Input: part model. Units: mm. Frame: model coordinates. A direction names the side the tool comes from. Round coordinates to 2 decimals unless told otherwise and drop trailing zeros. Order: outer loops, then holes, each group sorted by start corner. A loop starts at its lowest first (then second) coordinate and runs counter-clockwise, first axis right, second up. Notation, with made-up numbers: (53, -3) - (58, -3) arc R23 ccw to (58, 30) - close; hole circle Ø9 at (63.25, -9). An arc over 180 degrees is marked (long way). One line per item, written item: value. Start each with the question number.
from build123d import *

# Parameters (mm, degrees)
SKIZZE1_R                       = 30
AUFSATZ_LINEAR_AUSTRAGEN1_DEPTH = 30
SKIZZE2_R                       = 7.5
AUFSATZ_LINEAR_AUSTRAGEN2_DEPTH = 40
KREISMUSTER1_COUNT              = 8


with BuildPart() as part:
    # Skizze1 → Aufsatz-Linear austragen1 (new body)
    with BuildSketch(Plane.XY):
        Circle(SKIZZE1_R)
    extrude(amount=AUFSATZ_LINEAR_AUSTRAGEN1_DEPTH)

    # Skizze2 → Aufsatz-Linear austragen2 (add)
    with BuildSketch(Plane(origin=(0, 0, 0), x_dir=(1, 0, 0), z_dir=(0, 1, 0))):
        with Locations(Location((0, -15, 0), (0, 0, 90))):
            Circle(SKIZZE2_R)
    aufsatz_linear_austragen2 = extrude(amount=AUFSATZ_LINEAR_AUSTRAGEN2_DEPTH)

    # Kreismuster1: Aufsatz-Linear austragen2 ×8 about axis
    kreismuster1_axis = Axis((0, 0, 0), (0, 0, 1))
    for i in range(1, KREISMUSTER1_COUNT):
        add(aufsatz_linear_austragen2.rotate(kreismuster1_axis, i * 360 / KREISMUSTER1_COUNT))


solid = part.part
Item 1: Pull-direction query (Y, two-part tool) for faces 1 (the face through (0, 40, 15)), 2 (the face through (0, -40, 15)), 3 (the face through (19.099, 29.616, 15.976)); classes: released by +Y, released by -Y, zero draft, split by the parting line, or undercut.
Item 2: Line query: L1, parallel to Y at x = 26, z = 8.5; L2, parallel to Z at x = -33, y = 0.5; L3, parallel to Y at x = -9, z = 24.5. Output: solid intervals per line, ascending.
Item 3: Section query D-D on x = -13.5. Return loops of the section in (y, z), and give its area (3 significant figures).
Item 4: Section query A-A on y = 0. Return loops of the section in (x, z).
Item 5: Reachability of faces 4 (the face through (-34.447, -7.436, 15.976)), 5 (the face through (27.712, -11.49, 14.79)), 6 (the face through (34.447, 7.436, 15.976)) from +Z, -Z, +X, -X, +Y, -Y: full face, straight path, thin tool, end or side. Return the list, or none.
Item 6: First-contact query: pin 1 Ø5 at (y, z) = (-7, 8.5) entering from -X; pin 2 Ø3 at (x, z) = (24.5, 22.5) entering from -Y; pin 3 Ø5 at (x, y) = (-30, -20) entering from +Z. Flat tips, straight axial feed; report the tip coordinate or a pass-through.
Geometry results:
1. face 1: released by +Y
1. face 2: released by -Y
1. face 3: undercut
2. L1: y = -30.57 to -20.71, -14.97 to 14.97, 20.71 to 30.57
2. L2: z = 7.52 to 22.48
2. L3: y = -28.62 to 28.62
3. outline: (-26.79, 0) - (26.79, 0) - (26.79, 30) - (-26.79, 30) - close
3. area: 1,610 mm^2
4. outline: (-40, 7.5) - (-30, 7.5) - (-30, 0) - (30, 0) - (30, 7.5) - (40, 7.5) - (40, 22.5) - (30, 22.5) - (30, 30) - (-30, 30) - (-30, 22.5) - (-40, 22.5) - close
5. face 4: -X
5. face 5: none
5. face 6: +X
6. pin 1: stops at x = -40
6. pin 2: stops at y = -31.22
6. pin 3: stops at z = 20.95
